Input: part model. Units: mm. Frame: model coordinates. Face numbers are marked on the shaded views. A direction names the side the tool comes from. Give positions to 0.01 mm unless a question says otherwise; leave off trailing zeros. Loops run counter-clockwise (first coordinate to the right, second up) from the corner with the lowest first, then second, coordinate; pieces in that order, holes last. Notation, with made-up numbers: M 0,61.5 L 43,61.5 A28 ccw 43,79.5 Z; hole C 60,-25 d6. An arc over 180 degrees is marked long. Return JSON: item names as keys, results as strings. Group by question number.
```python
from build123d import *

# Parameters (mm, degrees)
SKETCH1_R           = 6.5
SKETCH1_R_2         = 1
BOSS_EXTRUDE1_DEPTH = 4
CUT_EXTRUDE2_DEPTH  = 5
CIRPATTERN2_COUNT   = 12
SKETCH11_R          = 4.5
BOSS_EXTRUDE2_DEPTH = 11
CUT_EXTRUDE3_START  = 11
CUT_EXTRUDE3_DEPTH  = 2
SKETCH13_R          = 1.9
CUT_EXTRUDE4_DEPTH  = 12


with BuildPart() as part:
    # Sketch1 → Boss-Extrude1 (new body)
    with BuildSketch(Plane.XY):
        Circle(SKETCH1_R)
        Circle(SKETCH1_R_2, mode=Mode.SUBTRACT)
    extrude(amount=BOSS_EXTRUDE1_DEPTH)

    # Sketch4 → Cut-Extrude2 (cut, through all)
    with BuildSketch(Plane.XY):
        with BuildLine():
            ThreePointArc((-0.500194414, 4.472114215), (0, 4.5), (0.500194414, 4.472114215))
            ThreePointArc((0.500194414, 4.472114215), (1.113314535, 5.941215952), (2.604960982, 6.497243899))
            ThreePointArc((2.604960982, 6.497243899), (0, 7), (-2.604960982, 6.497243899))
            ThreePointArc((-2.604960982, 6.497243899), (-1.123395838, 5.950848366), (-0.5, 4.5))
            ThreePointArc((-0.5, 4.5), (-0.500048604, 4.486056768), (-0.500194414, 4.472114215))
        make_face()
    cut_extrude2 = extrude(amount=CUT_EXTRUDE2_DEPTH, mode=Mode.SUBTRACT)

    # CirPattern2: Cut-Extrude2 ×12 about axis
    cirpattern2_axis = Axis((0, 0, 0), (0, 0, 1))
    for i in range(1, CIRPATTERN2_COUNT):
        add(cut_extrude2.rotate(cirpattern2_axis, i * 360 / CIRPATTERN2_COUNT), mode=Mode.SUBTRACT)

    # Sketch11 → Boss-Extrude2 (add)
    with BuildSketch(Plane.XY):
        Circle(SKETCH11_R)
    extrude(amount=BOSS_EXTRUDE2_DEPTH)

    # Sketch12 → Cut-Extrude3 (cut)
    with BuildSketch(Plane.XY.offset(CUT_EXTRUDE3_START)):
        Polygon((3.290896534, 0), (1.645448267, 2.85), (-1.645448267, 2.85), (-3.290896534, 0), (-1.645448267, -2.85), (1.645448267, -2.85), align=None)
    extrude(amount=-CUT_EXTRUDE3_DEPTH, mode=Mode.SUBTRACT)

    # Sketch13 → Cut-Extrude4 (cut, through all)
    with BuildSketch(Plane.XY):
        Circle(SKETCH13_R)
    extrude(amount=CUT_EXTRUDE4_DEPTH, mode=Mode.SUBTRACT)


solid = part.part
```
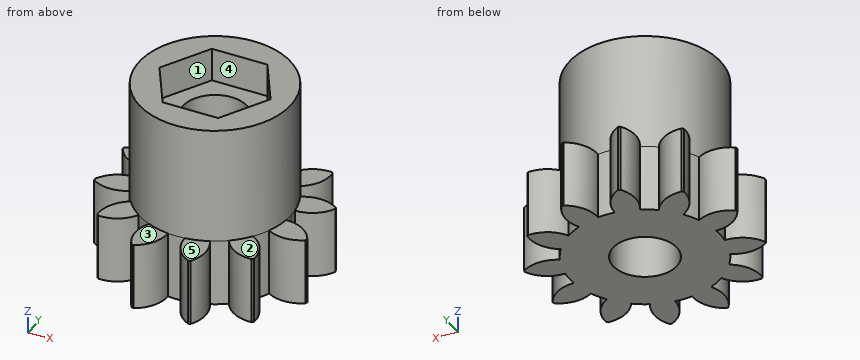
Item 1: Material intervals for line 1 (Y direction, x = 0, z = 6); line 2 (Y direction, x = 4, z = 3); line 3 (Z direction, x = 2, y = 0), sorted ascending. Write a range as from..to.
Item 2: Reachability of the marked faces 3, 4 and 5 from +Z, -Z, +X, -X, +Y, -Y: full face, straight path, thin tool, end or side. Return the list, or none.
Item 3: Section D-D, the plane y = 0.75. Return loops of the section in (x, z).
Item 4: Section C-C, the plane z = 5. Return loops of the section in (x, y), then the cut area to 3 significant figures.
Item 5: First-contact query: pin 1 Ø0.6 at (x, y) = (3.5, 4) entering from +Z; pin 2 Ø4 at (y, z) = (2, 7.5) entering from -X; pin 3 Ø0.6 at (x, z) = (0.5, 10) entering from -Y; pin 4 Ø1.7 at (x, y) = (-5, -1) entering from +Z. Flat tips, straight axial feed; report the tip coordinate or a pass-through.
Item 6: Section A-A, the plane x = 0. Return loops of the section in (y, z), then the cut area to 3 significant figures.
Item 7: Pull-direction query (Y, two-part tool) for the marked faces 1 and 2; classes: pulls with the +Y half, pulls with the -Y half, needs draft (parallel to the pull), parting line crosses it, or undercut.
Item 8: Section B-B, the plane y = 5.25. Return loops of the section in (x, z).
Answer below:
{
 "1": {"line 1": "-4.5..-1.9, 1.9..4.5", "line 2": "-4.6..-2.94, -2.06..2.06, 2.94..4.6", "line 3": "0..9"},
 "2": {"face 3": "+Z, -X, -Y", "face 4": "+Z", "face 5": "+Z, +X, -Y"},
 "3": {"outline": "M -5.47,0 L -1.75,0 L -1.75,9 L -2.86,9 L -2.86,11 L -4.44,11 L -4.44,4 L -5.47,4 Z; M 1.75,0 L 5.47,0 L 5.47,4 L 4.44,4 L 4.44,11 L 2.86,11 L 2.86,9 L 1.75,9 Z"},
 "4": {"outline": "C 0,0 d9; hole C 0,0 d3.8", "area": "52.3 mm^2"},
 "5": {"pin 1": "z = 4", "pin 2": "x = -4.5", "pin 3": "y = -4.5", "pin 4": "z = 11"},
 "6": {"outline": "M -4.5,0 L -1.9,0 L -1.9,9 L -2.85,9 L -2.85,11 L -4.5,11 Z; M 1.9,0 L 4.5,0 L 4.5,11 L 2.85,11 L 2.85,9 L 1.9,9 Z", "area": "53.4 mm^2"},
 "7": {"face 1": "undercut", "face 2": "needs draft"},
 "8": {"outline": "M -2.08,0 L -0.65,0 L -0.65,4 L -2.08,4 Z; M 0.65,0 L 2.08,0 L 2.08,4 L 0.65,4 Z"}
}
